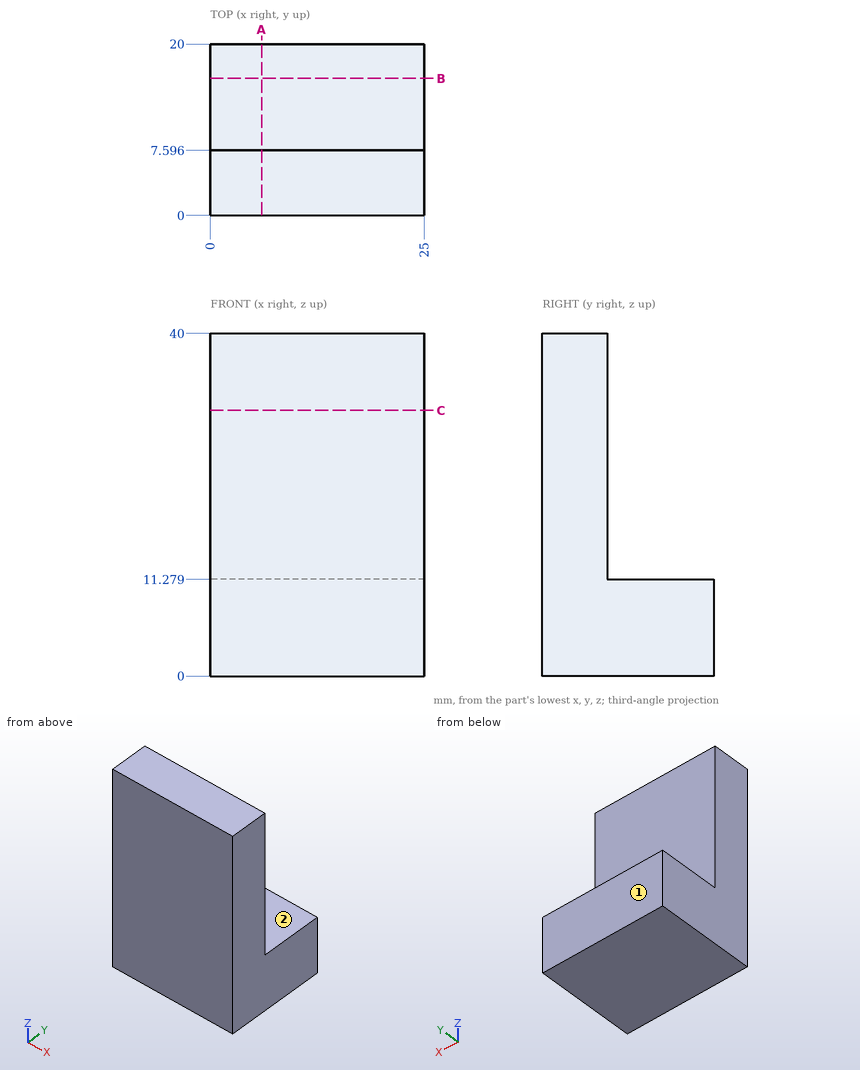
Geometry: see drawing. Coordinates: mm, zero at the bounding-box minimum. A direction names the side the tool comes from. Round coordinates to 2 decimals unless told otherwise and drop trailing zeros. Write each loop counter-clockwise with the first axis right and the second up, starting at its lowest first coordinate (ties: lowest second). Pieces come first, ordered by that corner, then holes.
1) Contact query for flat-ended pins moving along their axis: P1, Ø3.5, axis at x = 10.5, y = 17, coming from the +Z side; P2, Ø3, axis at x = 15.5, z = 23.5, coming from the +Y side. Output: stop coordinate, or through.
2) Reachability of the marked faces 1 and 2 from +Z, -Z, +X, -X, +Y, -Y: full face, straight path, thin tool, end or side. Return the list, or none.
3) Cut plane B-B (y = 16). Return the cut outline in (x, z), then the cut area to 3 significant figures.
4) Ray query, L1, parallel to Z at x = 3, y = 14.75; L2, parallel to Y at x = 19.25, z = 22. Return the intervals inside material, ascending.
5) Cut plane A-A (x = 6). Return the cut outline in (y, z).
6) Cut plane C-C (z = 31). Return the cut outline in (x, y).
Geometry says:
1. P1: stops at z = 11.28
1. P2: stops at y = 7.6
2. face 1: +Z, -Z, +X, -X, +Y
2. face 2: +Z, +X, -X, +Y
3. outline: (0, 0) - (25, 0) - (25, 11.28) - (0, 11.28) - close
3. area: 282 mm2
4. L1: z = 0 to 11.28
4. L2: y = 0 to 7.6
5. outline: (0, 0) - (20, 0) - (20, 11.28) - (7.6, 11.28) - (7.6, 40) - (0, 40) - close
6. outline: (0, 0) - (25, 0) - (25, 7.6) - (0, 7.6) - close
